Check sheet for the modelled part. Datum: model origin and axes. Units: mm. Face numbers are marked on the shaded views. A direction names the side the tool comes from. Give positions to 0.01 mm unless a question says otherwise; leave off trailing zeros. Loops run counter-clockwise (first coordinate to the right, second up) from the corner with the lowest first, then second, coordinate; pieces in that order, holes last. Notation, with made-up numbers: M 10,2 L 60,2 A31 ccw 60,31 Z; hole C -31,7.5 d1. An arc over 180 degrees is marked long. Put each result on its own line as item: value. Start each with the question number.
```python
from build123d import *

# Parameters (mm, degrees)
SKETCH_1_R          = 11.25
EXTRUDE_1_DEPTH     = 4
SKETCH_2_W          = 1.89000918
SKETCH_2_H          = 11.806467468
CUT_EXTRUDE_1_DEPTH = 2
EXTRUDE_2_DEPTH     = 20
EXTRUDE_3_DEPTH     = 2
CHAMFER_1_SIZE      = 3


with BuildPart() as part:
    # 草图1 → 凸台-拉伸1 (new body)
    with BuildSketch(Plane.XY):
        Circle(SKETCH_1_R)
    extrude(amount=EXTRUDE_1_DEPTH)

    # 草图2 → 切除-拉伸1 (cut)
    with BuildSketch(Plane.XY.offset(4)):
        Rectangle(SKETCH_2_W, SKETCH_2_H)
    extrude(amount=-CUT_EXTRUDE_1_DEPTH, mode=Mode.SUBTRACT)

    # 草图3 → 凸台-拉伸2 (add)
    with BuildSketch(Plane(origin=(0, 0, 0), x_dir=(-1, 0, 0), z_dir=(0, 0, -1))):
        with BuildLine():
            Line((-8.1, -3.923009049), (-8.1, 3.923009049))
            ThreePointArc((-8.1, 3.923009049), (0, 9), (8.1, 3.923009049))
            Line((8.1, 3.923009049), (8.1, -3.923009049))
            ThreePointArc((8.1, -3.923009049), (0, -9), (-8.1, -3.923009049))
        make_face()
    extrude(amount=EXTRUDE_2_DEPTH)

    # 草图4 → 凸台-拉伸3 (add)
    with BuildSketch(Plane(origin=(0, 0, -20), x_dir=(-1, 0, 0), z_dir=(0, 0, -1))):
        with BuildLine():
            Line((0, 5), (34, 5))
            ThreePointArc((34, 5), (39, 0), (34, -5))
            Line((34, -5), (0, -5))
            ThreePointArc((0, -5), (-5, 0), (0, 5))
        make_face()
    extrude(amount=EXTRUDE_3_DEPTH)

    # 倒角1
    chamfer_1_edges = [part.edges().sort_by_distance(p)[0] for p in [
        (-11.25, 0, 4),
    ]]
    chamfer(chamfer_1_edges, length=CHAMFER_1_SIZE)


solid = part.part
```
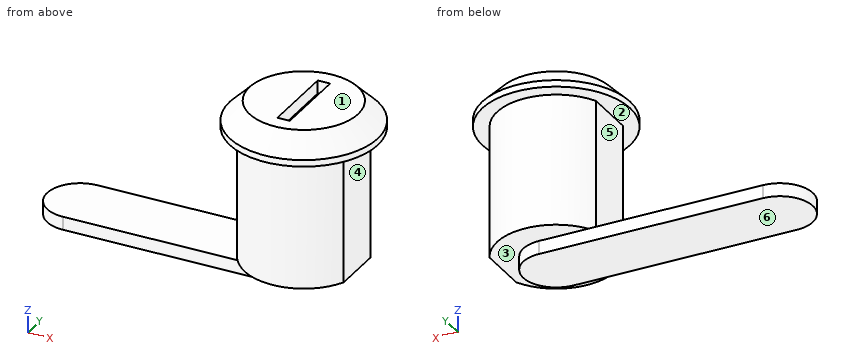
Q1. Mould release check, pull along Z, two halves, no side actions. Record for the marked faces 1, 2 and 3: pulls with the +Z half, pulls with the -Z half, needs draft (parallel to the pull), parting line crosses it, or undercut.
Q2. Depth check by flat-ended pin: P1, Ø8.5, axis at y = 0, z = -9, coming from the -X side; P2, Ø1, axis at x = -30.5, y = -6.5, coming from the -Z side; P3, Ø3, axis at x = -18, y = 0.5, coming from the +Z side; P4, Ø3, axis at y = 7, z = -13.5, coming from the +X side. Enter the tip coordinate at first touch or a pass-through.
Q3. Section check A-A, the plane y = 0. Record the cut outline in (x, z) (3 decimals), then the cut area to 3 significant figures.
Q4. Section check C-C, the plane z = -1.5. Record the cut outline in (x, y).
Q5. Access from +Z, -Z, +X, -X, +Y, -Y to the whole of each face (thin tool, end or side, straight path). Record for the marked faces 4, 5 and 6.
Q6. Thickness scan on line 1 along Z through (x, y) = (6.5, 3.25); line 2 along Z through (x, y) = (-13, -0.75); line 3 along X through (y, z) = (-3.5, -12.5). Record the ranges inside material, lowest first. Write a range as [from, to].
Q7. Section check B-B, the plane x = -16. Record the cut outline in (y, z), then the cut area to 3 significant figures.
Found:
1. face 1: pulls with the +Z half
1. face 2: undercut
1. face 3: pulls with the -Z half
2. P1: stops at x = -8.1
2. P2: passes through
2. P3: stops at z = -20
2. P4: stops at x = 7.12
3. outline: M -39,-22 L 5,-22 L 5,-20 L 8.1,-20 L 8.1,0 L 11.25,0 L 11.25,1 L 8.25,4 L 0.945,4 L 0.945,2 L -0.945,2 L -0.945,4 L -8.25,4 L -11.25,1 L -11.25,0 L -8.1,0 L -8.1,-20 L -39,-20 Z
3. area: 489 mm^2
4. outline: M -8.1,-3.92 A9 ccw 8.1,-3.92 L 8.1,3.92 A9 ccw -8.1,3.92 Z
5. face 4: -Z, +X, +Y, -Y
5. face 5: -X, +Y, -Y
5. face 6: -Z, +X, -X, +Y, -Y
6. line 1: z = [-20, 4]
6. line 2: z = [-22, -20]
6. line 3: x = [-8.1, 8.1]
7. outline: M -5,-22 L 5,-22 L 5,-20 L -5,-20 Z
7. area: 20.0 mm^2
